Part model, mm, in its own coordinate system. A direction names the side the tool comes from. Coordinates: 2 decimals unless noted, no trailing zeros. Loops run counter-clockwise (first coordinate to the right, second up) from the corner with the lowest first, then second, coordinate; pieces in that order, holes last. Notation, with made-up numbers: M -0.75,73.25 L 41.25,73.25 A3 cw 41.25,78.25 Z; hole C 69.25,20.25 d7. An arc over 180 degrees is marked long. Use a Markdown table: item, result. Add a question column.
1) Band-saw the part on D-D (y = 0). List the corners of the cut face in (x, z).
2) Pull direction Y, two halves, no side cores. Call faces 1 (the flat face through (0.6, -31, 35)), 2 (the flat face through (5.18, -32.49, 47.37)), 3 (the cylindrical face through (-13.058, -29.003, 35.49)): released by +Y, released by -Y, zero draft, split by the parting line, or undercut.
3) Tool access for faces 4 (the flat face through (5.18, -30.31, 47.37)), 5 (the cylindrical face through (-13.879, 30.673, 35.49)), 6 (the flat face through (5.18, -32.49, 22.63)), 7 (the flat face through (0, 2, 35)), 8 (the flat face through (10.5, -27, 35)): list every direction of +Z, -Z, +X, -X, +Y, -Y with a clear straight run to the whole face (end or side of a thin tool).
4) Band-saw the part on A-A (x = 7.75). List the corners of the cut face in (y, z), plus the area to 3 significant figures.
5) Band-saw the part on C-C (x = -6.75). List the corners of the cut face in (y, z), plus the area to 3 significant figures.
6) Pin check, flat tips, straight feed: pin 1 Ø3 at (x, z) = (-10, 62) entering from -Y; pin 2 Ø5 at (y, z) = (-20, 31) entering from -X; pin 3 Ø1.5 at (y, z) = (17.5, 13.5) entering from +X; pin 4 Ø2 at (y, z) = (-31.5, 40) entering from -X. Stop position of each tip, or through.
7) Wall check: probe 1 along X at (y, z) = (31.5, 8); probe 2 along Y at (x, z) = (6, 49); probe 3 along X at (y, z) = (-22, 23). Give the ranges that are in metal, low to high. Write a range as from..to.
8) Band-saw the part on B-B (y = -21). List the corners of the cut face in (x, z), plus the area to 3 significant figures.
from build123d import *

# Parameters (mm, degrees)
F0_W     = 9
F0_H     = 2.6991704602
F0_H_2   = 1.5
F1_DEPTH = 70
F2_R     = 1.55
F3_W     = 9.3
F3_H     = 22.7586206897
F4_DEPTH = 5
F5_SIZE  = 2
F6_R     = 0.59999
F7_R     = 1.6


# Not quite as in the source:
# - a fillet or chamfer is up to 0.001 mm smaller than in the source, because OpenCascade refuses the exact size
# - a feature names something its author has since deleted; it is built from what else it names


with BuildPart() as f1:
    # F0 (on Top) → F1 (new body)
    with BuildSketch(Plane.XY):
        Polygon((-9, -32), (-9, -29.3008295398), (-13.4364079285, -28.4836487781), (-13.9172762663, -31.0942438952), (-11.4586381331, -31.5471219476), align=None)
        with Locations((-4.5, -30.6504147699)):
            Rectangle(F0_W, F0_H)
        Polygon((-9, -33.5), (-9, -32), (-9.2639088239, -33.5), align=None)
        with Locations((-4.5, -32.75)):
            Rectangle(F0_W, F0_H_2)
        Polygon((-11.6319159151, -32.5319949396), (-11.4586381331, -31.5471219476), (-13.9172762663, -31.0942438952), align=None)
        with BuildLine():
            Line((0, -29.3008295398), (0, 29.3008295398))
            Line((0, 29.3008295398), (-9, 29.3008295398))
            ThreePointArc((-9, 29.3008295398), (-2.9680403173, 0), (-9, -29.3008295398))
            Line((-9, -29.3008295398), (0, -29.3008295398))
        make_face()
        with Locations((-4.5, 30.6504147699)):
            Rectangle(F0_W, F0_H)
        Polygon((0, 32), (0, 33.5), (-8.7112760279, 33.5), (-9, 32), align=None)
        Polygon((-9, 29.3008295398), (-9, 32), (-11.4586381331, 32.4528780524), (-13.9172762663, 32.9057561048), (-14.398144604, 30.2951609877), align=None)
        Polygon((-13.9172762663, 32.9057561048), (-11.4586381331, 32.4528780524), (-11.2696250671, 33.4348526248), align=None)
        Polygon((10.5, -29.3008295398), (0, -29.3008295398), (0, -32), (0, -33.5), (13.4, -33.5), (13.4, -15.5), (10.7962751514, -15.5), (10.5, -15.9545544746), (10.5, -22.238118574), (10.5, -25.2114422619), align=None)
        Polygon((10, -23.3806278557), (10.5, -25.2114422619), (10.5, -22.238118574), (10.5, -15.9545544746), (10, -16.7216698947), align=None)
    extrude(amount=F1_DEPTH)

    # F2
    f2_edges = [f1.edges().sort_by_distance(p)[0] for p in [
        (-14.398145, 30.295161, 35),
        (-9, 29.30083, 35),
        (-13.436408, -28.483649, 35),
        (-9, -29.30083, 35),
        (-13.917276, -31.094244, 35),
        (-13.917276, 32.905756, 35),
    ]]
    fillet(f2_edges, radius=F2_R)

    # F3 (on face) → F4 (cut)
    with BuildSketch(Plane.XZ.offset(33.5)):
        with Locations((5.25, 35)):
            Rectangle(F3_W, F3_H)
    extrude(amount=-F4_DEPTH, mode=Mode.SUBTRACT)

    # F5
    f5_edges = [f1.edges().sort_by_distance(p)[0] for p in [
        (5.25, -33.5, 46.37931),
        (5.25, -33.5, 23.62069),
        (5.25, -29.30083, 23.62069),
        (5.25, -29.30083, 46.37931),
    ]]
    chamfer(f5_edges, length=F5_SIZE)

    # F6 (radius 0.6 in the source; OpenCascade refuses exactly that, so slightly less here)
    f6_edges = [f1.edges().sort_by_distance(p)[0] for p in [
        (0, -29.30083, 35),
        (10.5, -29.30083, 35),
    ]]
    fillet(f6_edges, radius=F6_R)

    # F7
    f7_edges = [f1.edges().sort_by_distance(p)[0] for p in [
        (10.796275, -15.5, 35),
        (13.4, -15.5, 35),
        (10, -16.72167, 35),
        (13.4, -33.5, 35),
    ]]
    fillet(f7_edges, radius=F7_R)


solid = f1.part
Entries:
| question | item | result |
|---|---|---|
| 1 | outline | M -2.97,0 L 0,0 L 0,70 L -2.97,70 Z |
| 2 | face 1 | zero draft |
| 2 | face 2 | released by -Y |
| 2 | face 3 | undercut |
| 3 | face 4 | +Y |
| 3 | face 5 | +Z, -Z, -X |
| 3 | face 6 | -Y |
| 3 | face 7 | +Z, -Z, +Y |
| 3 | face 8 | +Z, -Z |
| 4 | outline | M -33.5,0 L -29.3,0 L -29.3,21.62 L -31.3,23.62 L -31.5,23.62 L -33.5,21.62 Z; M -33.5,48.38 L -31.5,46.38 L -31.3,46.38 L -29.3,48.38 L -29.3,70 L -33.5,70 Z |
| 4 | area | 190 mm2 |
| 5 | outline | M -33.5,0 L -23.38,0 L -23.38,70 L -33.5,70 Z; M 23.38,0 L 33.5,0 L 33.5,70 L 23.38,70 Z |
| 5 | area | 1,420 mm2 |
| 6 | pin 1 | y = -33.5 |
| 6 | pin 2 | x = -6.46 |
| 6 | pin 3 | x = 0 |
| 6 | pin 4 | x = -13.74 |
| 7 | probe 1 | -14.14..0 |
| 7 | probe 2 | -33.5..-29.3 |
| 7 | probe 3 | -6.31..0, 10..13.4 |
| 8 | outline | M -6,0 L 0,0 L 0,70 L -6,70 Z; M 10,0 L 13.4,0 L 13.4,70 L 10,70 Z |
| 8 | area | 658 mm2 |
